Part print with two shaded views. Sizes in mm from the minimum x, y, z corner. Coordinates: 2 decimals unless noted, no trailing zeros.
(1) Slice it at C-C (y = 1). Give the number of separate pieces and of enclosed holes in the cut face, and give its area (3 significant figures).
(2) Flat gauge pins, fed straight in: P1, Ø2, axis at x = 66.5, y = 5, coming from the +Z side; P2, Ø3, axis at y = 5.5, z = 83.5, coming from the -X side. Where does each tip first touch, or does it go through?
(3) Wall check: L1, parallel to Z at x = 25.5, y = 4.25 (1 decimal); L2, parallel to X at y = 4, z = 37 (1 decimal); L3, parallel to Z at x = 76, y = 6 (1 decimal). Give the ranges that are in metal, low to high.
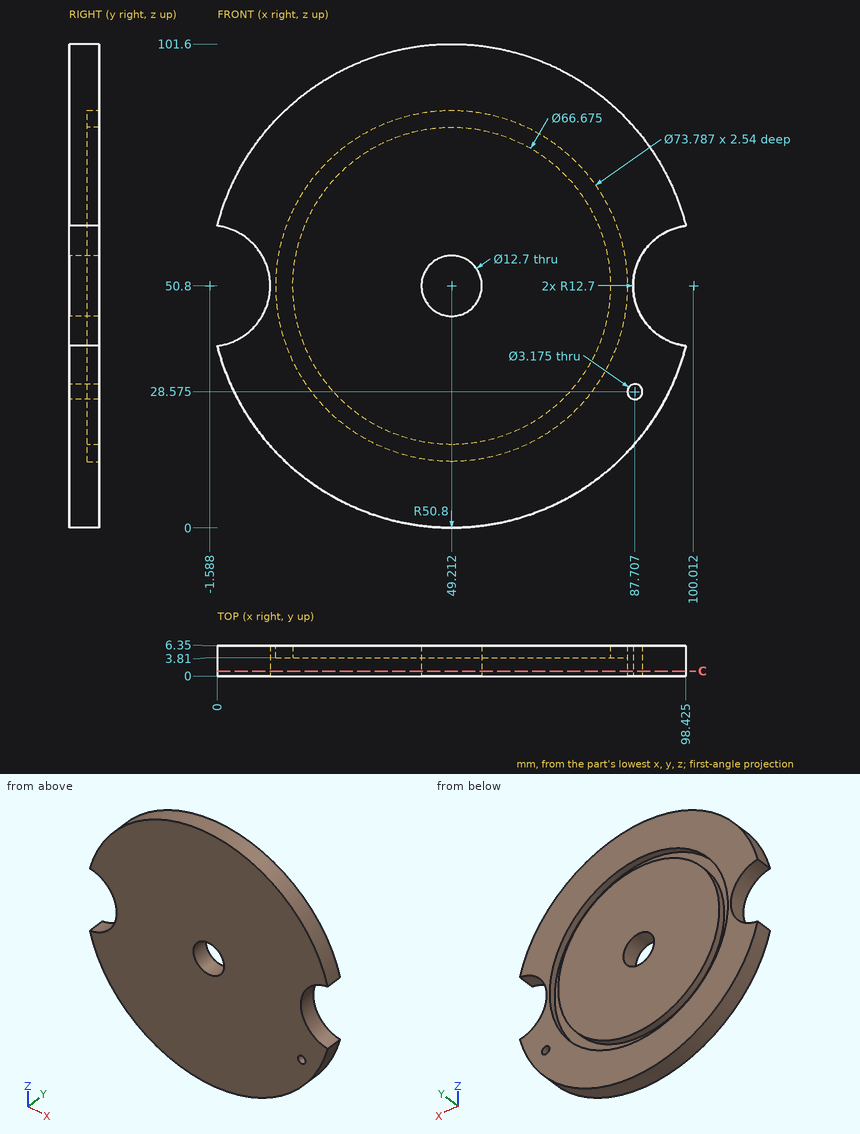
Response values:
1. separate pieces: 1
1. enclosed holes: 2
1. area: 7,490 mm2
2. P1: stops at z = 98.92
2. P2: stops at x = 9.12
3. L1: z = 5.9 to 22.5, 27.4 to 74.2, 79.1 to 95.7
3. L2: x = 0.3 to 15, 18.9 to 79.6, 83.4 to 98.1
3. L3: z = 7.6 to 25.4, 31 to 70.6, 76.2 to 94
